Model file for the job. Use its own axes, mm. A direction names the side the tool comes from. Round coordinates to 2 decimals unless told otherwise and drop trailing zeros. Loops run counter-clockwise (first coordinate to the right, second up) from the corner with the lowest first, then second, coordinate; pieces in that order, holes last. Notation, with made-up numbers: (-34.5, -32) -> (15.5, -32) arc R16 ccw to (15.5, -1) -> close; hole circle Ø3 at (-22, 23.5). An arc over 180 degrees is marked (long way). Use a Markdown table: item, result.
Autodesk Inventor part; units mm, degrees
ref_plane "YZ Plane" through (0, 0, 0) normal (1, 0, 0) x (0, 1, 0)
ref_plane "XZ Plane" through (0, 0, 0) normal (0, 1, 0) x (-1, 0, 0)
ref_plane "XY Plane" through (0, 0, 0) normal (0, 0, 1) x (1, 0, 0)
sketch "Sketch1" plane through (0, 0, 0) normal (0, 1, 0) x (-1, 0, 0)
  line L0 (-9.35, 0) -> (-9.35, -12.5) construction
  line L1 (-25.4, 0) -> (-25.4, -12.5) construction
  line L2 (-9.35, -6.9) -> (-25.4, -6.9)
  line L3 (-25.4, -6.9) -> (-25.4, -5.6)
  line L4 (-25.4, -5.6) -> (-9.35, -5.6)
  line L5 (-9.35, -5.6) -> (-9.35, -6.9)
  circle A0 centre (-4.875, -6.25) radius 1
  circle A1 centre (-29.875, -6.25) radius 1
  line L6 (-9.35, 0) -> (-8.9, 0) construction
  line L7 (-25.4, 0) -> (-25.85, 0) construction
  line L8 (-8.45, -10.4049) -> (-8.45, -12.05)
  line L9 (-9.35, -12.05) -> (-9.35, -0.45)
  arc A2 (-8.45, -0.45) -> (-9.35, -0.45) centre (-8.9, -0.45) ccw
  arc A3 (-9.35, -12.05) -> (-8.45, -12.05) centre (-8.9, -12.05) ccw
  line L10 (-25.4, -12.05) -> (-25.4, -0.45)
  arc A4 (-25.4, -0.45) -> (-26.3, -0.45) centre (-25.85, -0.45) ccw
  arc A5 (-26.3, -12.05) -> (-25.4, -12.05) centre (-25.85, -12.05) ccw
  line L11 (-6.8219, -9.8759) -> (-4.9877, -12.4004)
  line L12 (-4.2596, -11.8714) -> (-5.0989, -10.7162)
  arc A6 (-4.9877, -12.4004) -> (-4.2596, -11.8714) centre (-4.6236, -12.1359) ccw
  line L13 (-3.9482, -9.3926) -> (-0.6086, -11.1683)
  line L14 (-0.1861, -10.3736) -> (-1.7142, -9.5611)
  arc A7 (-0.6086, -11.1683) -> (-0.1861, -10.3736) centre (-0.3973, -10.771) ccw
  line L15 (-1.3864, -8.7291) -> (-0.5511, -8.9529)
  line L16 (-0.3182, -8.0836) -> (-8.3489, -5.9318)
  arc A8 (-0.5511, -8.9529) -> (-0.3182, -8.0836) centre (-0.4347, -8.5183) ccw
  arc A9 (-6.8219, -9.8759) -> (-8.45, -10.4049) centre (-7.55, -10.4049) ccw
  arc A10 (-3.9482, -9.3926) -> (-5.0989, -10.7162) centre (-4.3708, -10.1872) ccw
  arc A11 (-1.3864, -8.7291) -> (-1.7142, -9.5611) centre (-1.5029, -9.1638) ccw
  line L17 (-8.45, -2.0951) -> (-8.45, -0.45)
  line L18 (-6.8219, -2.6241) -> (-4.9877, -0.0996)
  line L19 (-4.2596, -0.6286) -> (-5.0989, -1.7838)
  arc A12 (-4.2596, -0.6286) -> (-4.9877, -0.0996) centre (-4.6236, -0.3641) ccw
  line L20 (-3.9482, -3.1074) -> (-0.6086, -1.3317)
  line L21 (-0.1861, -2.1264) -> (-1.7142, -2.9389)
  arc A13 (-0.1861, -2.1264) -> (-0.6086, -1.3317) centre (-0.3973, -1.729) ccw
  line L22 (-1.3864, -3.7709) -> (-0.5511, -3.5471)
  line L23 (-0.3182, -4.4164) -> (-8.3489, -6.5682)
  arc A14 (-0.3182, -4.4164) -> (-0.5511, -3.5471) centre (-0.4347, -3.9817) ccw
  arc A15 (-8.45, -2.0951) -> (-6.8219, -2.6241) centre (-7.55, -2.0951) ccw
  arc A16 (-5.0989, -1.7838) -> (-3.9482, -3.1074) centre (-4.3708, -2.3128) ccw
  arc A17 (-1.7142, -2.9389) -> (-1.3864, -3.7709) centre (-1.5029, -3.3362) ccw
  line L24 (-26.3, -10.4049) -> (-26.3, -12.05)
  arc A18 (-26.3, -12.05) -> (-25.4, -12.05) centre (-25.85, -12.05) ccw
  line L25 (-27.9281, -9.8759) -> (-29.7623, -12.4004)
  line L26 (-30.4904, -11.8714) -> (-29.6511, -10.7162)
  arc A19 (-30.4904, -11.8714) -> (-29.7623, -12.4004) centre (-30.1264, -12.1359) ccw
  line L27 (-30.8018, -9.3926) -> (-34.1414, -11.1683)
  line L28 (-34.5639, -10.3736) -> (-33.0358, -9.5611)
  arc A20 (-34.5639, -10.3736) -> (-34.1414, -11.1683) centre (-34.3527, -10.771) ccw
  line L29 (-33.3636, -8.7291) -> (-34.1989, -8.9529)
  line L30 (-34.4318, -8.0836) -> (-26.4011, -5.9318)
  arc A21 (-34.4318, -8.0836) -> (-34.1989, -8.9529) centre (-34.3153, -8.5183) ccw
  arc A22 (-26.3, -10.4049) -> (-27.9281, -9.8759) centre (-27.2, -10.4049) ccw
  arc A23 (-29.6511, -10.7162) -> (-30.8018, -9.3926) centre (-30.3792, -10.1872) ccw
  arc A24 (-33.0358, -9.5611) -> (-33.3636, -8.7291) centre (-33.2471, -9.1638) ccw
  line L31 (-26.3, -2.0951) -> (-26.3, -0.45)
  arc A25 (-27.9281, -2.6241) -> (-26.3, -2.0951) centre (-27.2, -2.0951) ccw
  line L32 (-27.9281, -2.6241) -> (-29.7623, -0.0996)
  arc A26 (-29.7623, -0.0996) -> (-30.4904, -0.6286) centre (-30.1264, -0.3641) ccw
  line L33 (-30.4904, -0.6286) -> (-29.6511, -1.7838)
  arc A27 (-30.8018, -3.1074) -> (-29.6511, -1.7838) centre (-30.3792, -2.3128) ccw
  line L34 (-30.8018, -3.1074) -> (-34.1414, -1.3317)
  arc A28 (-34.1414, -1.3317) -> (-34.5639, -2.1264) centre (-34.3527, -1.729) ccw
  line L35 (-34.5639, -2.1264) -> (-33.0358, -2.9389)
  arc A29 (-33.3636, -3.7709) -> (-33.0358, -2.9389) centre (-33.2471, -3.3362) ccw
  line L36 (-33.3636, -3.7709) -> (-34.1989, -3.5471)
  arc A30 (-34.1989, -3.5471) -> (-34.4318, -4.4164) centre (-34.3153, -3.9817) ccw
  line L37 (-34.4318, -4.4164) -> (-26.4011, -6.5682)
  point P0 (0, 0)
  point P1 (-25.85, -6.25)
  point P2 (-6.6296, -9.375)
  point P3 (-4.45, -8.6161)
  point P4 (-4.45, -7.4424)
  point P5 (-30.5005, -5.4698)
  point P6 (-30.5005, -7.0302)
  point P7 (-4.2495, -7.0302)
  point P8 (-4.2495, -5.4698)
extrude "Extrusion1" add sketch "Sketch1" along normal blind 38 contours L2 L3 L4 L5 | L5 L9 A2 L17 A15 L18 A12 L19 A16 L20 A13 L21 A17 L22 A14 L23 A0 L16 A8 L15 A11 L14 A7 L13 A10 L12 A6 L11 A9 L8 A3 | L10 A5 L24 A22 L25 A19 L26 A23 L27 A20 L28 A24 L29 A21 L30 A1 L37 A30 L36 A29 L35 A28 L34 A27 L33 A26 L32 A25 L31 A4 L3 | L16 L23 A0 | A1 L37 L30 picked at (-6.2987, -6.25) picked at (-28.4488, -6.2912)
extrude "Extrusion2" add sketch "Sketch1" along normal blind 8 and the other way blind 4 contours L16 A0 L23 | A0 L16 | L30 A1 | A1 L37 L30 | L23 A0 | A1 L37 picked at (-4.6521, -6.705) picked at (-30.1259, -6.0659)
sketch "Sketch2" plane through (9.35, 0, -5.6) normal (0, 0, 1) x (1, 0, 0)
  line L0 (0, 0) -> (16.05, 0) construction
  line L1 (8.025, 0) -> (13.525, 0) construction
  line L2 (13.525, 0) -> (2.525, 0)
  line L3 (2.525, 0) -> (2.525, 9.3)
  line L4 (2.525, 9.3) -> (13.525, 9.3)
  line L5 (13.525, 9.3) -> (13.525, 0)
  line L6 (0, 38) -> (16.05, 38) construction
  circle A0 centre (8.025, 25.5) radius 1.5
  circle A1 centre (8.025, 18.5) radius 1.5
  circle A2 centre (8.025, 13.5) radius 1.5
  point P0 (-9.35, 0)
extrude "Extrusion3" cut sketch "Sketch2" against normal through all
properties part number "Steren Heatsink" material "Aluminum 6061"
Q1. Band-saw the part on D-D, the plane x = 8.9. Give the cut face in (y, z), plus the area to 3 significant figures.
Results list:
| item | result |
|---|---|
| outline | (0, -12.5) -> (38, -12.5) -> (38, 0) -> (0, 0) -> close |
| area | 475 mm² |
Q2. Tool access for faces 1 (the face through (16.269, 19.514, -6.241)), 2 (the face through (4.673, 18.734, -11.302)), 3 (the face through (32.45, 18.73, -2.23)), 4 (the face through (5, 8, -6)), 5 (the face through (26.3, 19, -11)): list every direction of +Z, -Z, +X, -X, +Y, -Y with a clear straight run to the whole face (end or side of a thin tool).
Results list:
| item | result |
|---|---|
| face 1 | +Z, -Z |
| face 2 | +Y, -Y |
| face 3 | +Z, +Y, -Y |
| face 4 | +Y |
| face 5 | -Z, +Y, -Y |
Q3. Pull direction X, two halves, no side cores. Call faces 6 (the face through (26.3, 19, -1)), 7 (the face through (5, -4, -6)): released by +X, released by -X, zero draft, split by the parting line, or undercut.
Results list:
| item | result |
|---|---|
| face 6 | undercut |
| face 7 | zero draft |
Q4. Flat gauge pins, fed straight in: pin 1 (0.8 mm diameter, centred on y = 24.5, z = -1.5, fed in from -X); pin 2 (1.4 mm diameter, centred on x = 15.5, z = -6.5, fed in from -Y); pin 3 (1.5 mm diameter, centred on y = 14, z = -9.5, fed in from +X); pin 4 (1 mm diameter, centred on x = 10, z = -6, fed in from -Y). Where does each tip first touch, or does it go through?
Results list:
| item | result |
|---|---|
| pin 1 | stops at x = -0.05 |
| pin 2 | stops at y = 9.3 |
| pin 3 | stops at x = 34.7 |
| pin 4 | stops at y = 0 |
Q5. Band-saw the part on B-B, the plane x = 17. Give the cut face in (y, z).
Results list:
| item | result |
|---|---|
| outline | (9.3, -6.9) -> (12.05, -6.9) -> (12.05, -5.6) -> (9.3, -5.6) -> close; (14.95, -6.9) -> (17.05, -6.9) -> (17.05, -5.6) -> (14.95, -5.6) -> close; (19.95, -6.9) -> (24.05, -6.9) -> (24.05, -5.6) -> (19.95, -5.6) -> close; (26.95, -6.9) -> (38, -6.9) -> (38, -5.6) -> (26.95, -5.6) -> close |
Q6. Band-saw the part on A-A, the plane z = -6.25. Give the cut face in (x, y) (3 decimals), plus the area to 3 significant figures.
Results list:
| item | result |
|---|---|
| outline | (3.875, -4) -> (5.875, -4) -> (5.875, 0) -> (11.875, 0) -> (11.875, 9.3) -> (22.875, 9.3) -> (22.875, 0) -> (28.875, 0) -> (28.875, -4) -> (30.875, -4) -> (30.875, 8) -> (28.875, 8) -> (28.875, 38) -> (5.875, 38) -> (5.875, 8) -> (3.875, 8) -> close; hole circle Ø3 at (17.375, 13.5); hole circle Ø3 at (17.375, 18.5); hole circle Ø3 at (17.375, 25.5) |
| area | 798 mm² |
Q7. Drill centre lines: L1, parallel to X at y = 7.5, z = -4; L2, parallel to X at y = 18, z = -1; L3, parallel to Z at x = 14, y = 36. Where is each one in solid material? Low to high. Write a range as from..to.
Results list:
| item | result |
|---|---|
| L1 | x = -0.01..9.35, 25.4..34.76 |
| L2 | x = 4.53..5.64, 8.45..9.35, 25.4..26.3, 29.11..30.22 |
| L3 | z = -6.9..-5.6 |
Q8. Band-saw the part on C-C, the plane x = 3. Give the cut face in (y, z), plus the area to 3 significant figures.
Results list:
| item | result |
|---|---|
| outline | (0, -9.9) -> (38, -9.9) -> (38, -7.37) -> (0, -7.37) -> close; (0, -5.13) -> (38, -5.13) -> (38, -2.6) -> (0, -2.6) -> close |
| area | 192 mm² |
